Check sheet for the modelled part. Datum: model origin and axes. Units: mm. Face numbers are marked on the shaded views. A direction names the side the tool comes from. Give positions to 0.01 mm unless a question says otherwise; leave off trailing zeros. Loops run counter-clockwise (first coordinate to the right, second up) from the corner with the lowest first, then second, coordinate; pieces in that order, holes last. Notation, with made-up numbers: M 63,-21 L 82,-21 A33 ccw 82,15 Z; hole C -2.75,28.5 d2. An arc over 180 degrees is marked long. One line per question, with ' | ' between items. Start each with the question number.
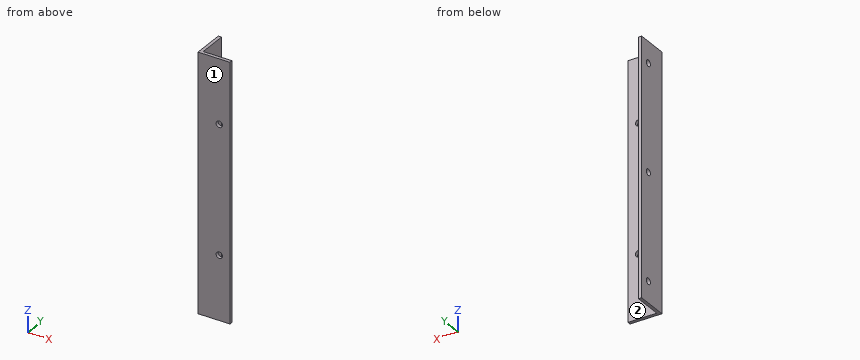
from build123d import *

# Parameters (mm, degrees)
EXTRUSION1_DEPTH               = 120
ESQUISSE2_R                    = 1.5
EXTRUSION2_DEPTH               = 122.86057607
ESQUISSE3_R                    = 1.5
EXTRUSION3_DEPTH               = 120
R_P_TITION_LIN_AIRE1_COUNT     = 2
R_P_TITION_LIN_AIRE1_PITCH     = 60
R_P_TITION_LIN_AIRE2_COUNT     = 2
R_P_TITION_LIN_AIRE2_PITCH     = 50
R_P_TITION_LIN_AIRE2_COL_COUNT = 2
R_P_TITION_LIN_AIRE2_COL_PITCH = 50


with BuildPart() as part:
    # Esquisse1 → Extrusion1 (new body)
    with BuildSketch(Plane.XY):
        Polygon((0, 0), (1.5, 0), (15, 0), (15, 1.5), (1.5, 1.5), (1.5, 15), (0, 15), align=None)
    extrude(amount=EXTRUSION1_DEPTH)

    # Esquisse2 → Extrusion2 (cut, through all)
    with BuildSketch(Plane.ZY):
        with Locations((60, 10)):
            Circle(ESQUISSE2_R)
    extrusion2 = extrude(amount=-EXTRUSION2_DEPTH, mode=Mode.SUBTRACT)

    # Esquisse3 → Extrusion3 (cut)
    with BuildSketch(Plane.XZ):
        with Locations(Location((10, 90, 0), (0, 0, 270))):
            Circle(ESQUISSE3_R)
    extrusion3 = extrude(amount=-EXTRUSION3_DEPTH, mode=Mode.SUBTRACT)

    # R_p_tition lin_aire1: Extrusion3 ×2
    with Locations(*[(0, 0, -i * R_P_TITION_LIN_AIRE1_PITCH) for i in range(1, R_P_TITION_LIN_AIRE1_COUNT)]):
        add(extrusion3, mode=Mode.SUBTRACT)

    # R_p_tition lin_aire2: Extrusion2 ×2
    with Locations(*[(0, 0, i * R_P_TITION_LIN_AIRE2_PITCH) for i in range(1, R_P_TITION_LIN_AIRE2_COUNT)]):
        add(extrusion2, mode=Mode.SUBTRACT)

    # R_p_tition lin_aire2 col: Extrusion2 ×2
    with Locations(*[(0, 0, -i * R_P_TITION_LIN_AIRE2_COL_PITCH) for i in range(1, R_P_TITION_LIN_AIRE2_COL_COUNT)]):
        add(extrusion2, mode=Mode.SUBTRACT)


solid = part.part
Q1. Depth check by flat-ended pin: P1, Ø3, axis at x = 5.5, y = 3.5, coming from the +Z side; P2, Ø4, axis at y = 10.5, z = 31.5, coming from the +X side; P3, Ø1.5, axis at x = 9.5, z = 91.5, coming from the +Y side. Enter the tip coordinate at first touch or a pass-through.
Q2. Cross-section at A-A (y = 10). Record the cut outline in (x, z).
Q3. Cross-section at D-D (z = 27). Record the cut outline in (x, y), and give its area (4 significant figures).
Q4. Cross-section at B-B (z = 10). Record the cut outline in (x, y), and give its area (4 significant figures).
Q5. Material ranges on probe 1 along Y at (x, z) = (1.1, 60); probe 2 along X at (y, z) = (6, 8), recorded low to high. Write a range as from..to.
Q6. Cross-section at C-C (x = 10). Record the cut outline in (y, z).
Q7. Access from +Z, -Z, +X, -X, +Y, -Y to the whole of each face (thin tool, end or side, straight path). Record for the marked faces 1 and 2.
Solved:
1) P1: passes through | P2: stops at x = 1.5 | P3: stops at y = 1.5
2) outline: M 0,0 L 1.5,0 L 1.5,8.5 L 0,8.5 Z; M 0,11.5 L 1.5,11.5 L 1.5,58.5 L 0,58.5 Z; M 0,61.5 L 1.5,61.5 L 1.5,108.5 L 0,108.5 Z; M 0,111.5 L 1.5,111.5 L 1.5,120 L 0,120 Z
3) outline: M 0,0 L 15,0 L 15,1.5 L 1.5,1.5 L 1.5,15 L 0,15 Z | area: 42.75 mm²
4) outline: M 0,0 L 15,0 L 15,1.5 L 1.5,1.5 L 1.5,8.5 L 0,8.5 Z; M 0,11.5 L 1.5,11.5 L 1.5,15 L 0,15 Z | area: 38.25 mm²
5) probe 1: y = 0..8.5, 11.5..15 | probe 2: x = 0..1.5
6) outline: M 0,0 L 1.5,0 L 1.5,28.5 L 0,28.5 Z; M 0,31.5 L 1.5,31.5 L 1.5,88.5 L 0,88.5 Z; M 0,91.5 L 1.5,91.5 L 1.5,120 L 0,120 Z
7) face 1: +Z, -Z, +X, -X, -Y | face 2: +Z, -Z, +X, +Y
